Verification items for the finished model (mm, model axes). Round coordinates to 2 decimals unless told otherwise and drop trailing zeros. Write each loop counter-clockwise with the first axis right and the second up, starting at its lowest first coordinate (ties: lowest second). Pieces come first, ordered by that corner, then holes. Notation, with made-up numbers: (25, -7.75) - (38, -7.75) arc R18 ccw to (38, 3.25) - close; hole circle Ø8 at (60, 63.5). An arc over 180 degrees is marked (long way). Answer as a JSON object with one key per item and string values.
```python
from build123d import *

# Parameters (mm, degrees)
SKETCH_1_R          = 40
SKETCH_1_R_2        = 5
EXTRUDE_1_DEPTH     = 20
FILLET_1_R          = 3
SKETCH_2_R          = 2.5
CUT_EXTRUDE_1_DEPTH = 61


with BuildPart() as part:
    # 草圖1 → 填料-伸長1 (new body)
    with BuildSketch(Plane(origin=(0, 0, 0), x_dir=(1, 0, 0), z_dir=(0, 1, 0))):
        with Locations(Location((0, 0, 0), (0, 0, 270))):
            Circle(SKETCH_1_R)
        with Locations(Location((0, 0, 0), (0, 0, 270))):
            Circle(SKETCH_1_R_2, mode=Mode.SUBTRACT)
    extrude(amount=EXTRUDE_1_DEPTH)

    # 圓角1
    fillet_1_edges = [part.edges().sort_by_distance(p)[0] for p in [
        (0, 0, -40),
        (0, 20, -40),
    ]]
    fillet(fillet_1_edges, radius=FILLET_1_R)

    # 草圖2 → 除料-伸長1 (cut, through all)
    with BuildSketch(Plane(origin=(0, 20, 0), x_dir=(1, 0, 0), z_dir=(0, 1, 0))):
        with Locations(Location((0, 20, 0), (0, 0, 270))):
            Circle(SKETCH_2_R)
        with Locations(Location((0, -20, 0), (0, 0, 270))):
            Circle(SKETCH_2_R)
    extrude(amount=-CUT_EXTRUDE_1_DEPTH, mode=Mode.SUBTRACT)


solid = part.part
```
1. Material ranges on probe 1 along X at (y, z) = (9.25, -20); probe 2 along X at (y, z) = (5, -18.5); probe 3 along Z at (x, y) = (31.5, 2), recorded low to high. Write a range as from..to.
Completed:
{"probe 1": "x = -34.64..-2.5, 2.5..34.64", "probe 2": "x = -35.46..-2, 2..35.46", "probe 3": "z = -24.37..24.37"}
2. Cross-section at B-B (x = 0). Record the boundary of the cut face in (y, z).
Completed:
{"outline": "(0, -37) arc R3 ccw to (3, -40) - (17, -40) arc R3 ccw to (20, -37) - (20, -22.5) - (0, -22.5) - close; (0, -17.5) - (20, -17.5) - (20, -5) - (0, -5) - close; (0, 5) - (20, 5) - (20, 17.5) - (0, 17.5) - close; (0, 22.5) - (20, 22.5) - (20, 37) arc R3 ccw to (17, 40) - (3, 40) arc R3 ccw to (0, 37) - close"}
3. Cross-section at A-A (z = 0). Record the boundary of the cut face in (x, y).
Completed:
{"outline": "(-40, 3) arc R3 ccw to (-37, 0) - (-5, 0) - (-5, 20) - (-37, 20) arc R3 ccw to (-40, 17) - close; (5, 0) - (37, 0) arc R3 ccw to (40, 3) - (40, 17) arc R3 ccw to (37, 20) - (5, 20) - close"}
4. Go/stop test with flat-tipped pins: pin 1 (6 mm diameter, centred on y = 3.5, z = 9.5, fed in from -X); pin 2 (1.5 mm diameter, centred on x = 30.5, y = 7.5, fed in from +Z); pin 3 (12 mm diameter, centred on x = -22, y = 5, fed in from +Z). Record where each tip stops, or that it passes through.
Completed:
{"pin 1": "stops at x = -39.47", "pin 2": "stops at z = 26.74", "pin 3": "stops at z = 36.66"}
5. Mould release check, pull along X, two halves, no side actions. Record for faces 1 (the face through (-8, 20, -1)), 2 (the face through (-39.05, 9.9, -8.67)), 3 (the face through (0.1, 10.1, -22.5)): released by +X, released by -X, zero draft, split by the parting line, or undercut.
Completed:
{"face 1": "zero draft", "face 2": "split by the parting line", "face 3": "undercut"}
